```python
from build123d import *

# Parameters (mm, degrees)
SKETCH1_W           = 18.923
SKETCH1_H           = 44.323
BOSS_EXTRUDE1_DEPTH = 63.5
FILLET1_R           = 3.175
SKETCH2_R           = 2.4892
CUT_EXTRUDE1_DEPTH  = 63.5
SKETCH3_R           = 2.4892
CUT_EXTRUDE2_DEPTH  = 63.5


with BuildPart() as part:
    # Sketch1 → Boss-Extrude1 (new body)
    with BuildSketch(Plane.XY):
        with Locations((9.4615, 22.1615)):
            Rectangle(SKETCH1_W, SKETCH1_H)
    extrude(amount=BOSS_EXTRUDE1_DEPTH)

    # Fillet1
    fillet1_edges = [part.edges().sort_by_distance(p)[0] for p in [
        (0, 44.323, 31.75),
        (18.923, 44.323, 31.75),
        (18.923, 0, 31.75),
        (0, 0, 31.75),
    ]]
    fillet(fillet1_edges, radius=FILLET1_R)

    # Sketch2 → Cut-Extrude1 (cut)
    with BuildSketch(Plane(origin=(0, 44.323, 0), x_dir=(1, 0, 0), z_dir=(0, 1, 0))):
        with Locations(Location((9.4615, -6.35, 0), (0, 0, 270))):
            Circle(SKETCH2_R)
        with Locations(Location((9.4615, -19.05, 0), (0, 0, 270))):
            Circle(SKETCH2_R)
        with Locations(Location((9.4615, -31.75, 0), (0, 0, 270))):
            Circle(SKETCH2_R)
        with Locations(Location((9.4615, -44.45, 0), (0, 0, 270))):
            Circle(SKETCH2_R)
        with Locations(Location((9.4615, -57.15, 0), (0, 0, 270))):
            Circle(SKETCH2_R)
    extrude(amount=-CUT_EXTRUDE1_DEPTH, mode=Mode.SUBTRACT)

    # Sketch3 → Cut-Extrude2 (cut)
    with BuildSketch(Plane(origin=(18.923, 0, 0), x_dir=(0, 0, -1), z_dir=(1, 0, 0))):
        with Locations(Location((-57.15, 34.8615, 0), (0, 0, 90))):
            Circle(SKETCH3_R)
        with Locations(Location((-44.45, 34.8615, 0), (0, 0, 90))):
            Circle(SKETCH3_R)
        with Locations(Location((-31.75, 34.8615, 0), (0, 0, 90))):
            Circle(SKETCH3_R)
        with Locations(Location((-19.05, 34.8615, 0), (0, 0, 90))):
            Circle(SKETCH3_R)
        with Locations(Location((-6.35, 34.8615, 0), (0, 0, 90))):
            Circle(SKETCH3_R)
        with Locations(Location((-44.45, 9.4615, 0), (0, 0, 90))):
            Circle(SKETCH3_R)
        with Locations(Location((-31.75, 9.4615, 0), (0, 0, 90))):
            Circle(SKETCH3_R)
        with Locations(Location((-19.05, 9.4615, 0), (0, 0, 90))):
            Circle(SKETCH3_R)
        with Locations(Location((-6.35, 9.4615, 0), (0, 0, 90))):
            Circle(SKETCH3_R)
        with Locations(Location((-57.15, 9.4615, 0), (0, 0, 90))):
            Circle(SKETCH3_R)
    extrude(amount=-CUT_EXTRUDE2_DEPTH, mode=Mode.SUBTRACT)


solid = part.part
```
Could you check a few things on this model? Use its own coordinates, in mm. Round coordinates to 2 decimals unless told otherwise and drop trailing zeros. Write each loop counter-clockwise with the first axis right and the second up, starting at its lowest first coordinate (ties: lowest second). Pieces come first, ordered by that corner, then holes. Notation, with made-up numbers: M 85.5,-23 L 117.5,-23 A22 cw 117.5,8 Z; hole C -24,39 d6. An arc over 180 degrees is marked long. Answer in a Markdown table with one row per item. Add a question column.
Q1. If we mould it in two halves opening along X, with no side actions, what happens to faces 1 (the cylindrical face through (7.95, 40.71, 17.07)), 2 (the cylindrical face through (15.31, 11.836, 7.098)), 3 (the cylindrical face through (0.905, 43.368, 32.194))? For each: +X half, -X half, draft (parallel to the pull), parting line (faces both ways), or undercut.
Q2. Will this pin go through, and if not, where does the flat tip stop? pin 1 Ø6.5 at (x, z) = (9.46, 31.75) entering from +Y.
Q3. Imagine slicing it at A-A (y = 18.5). Please give me the cut outline in (x, z).
Q4. If I drill on line 1 (Y direction, x = 13, z = 31.75); line 2 (X direction, y = 37.5, z = 19.05); line 3 (Y direction, x = 16.25, z = 30), over which ranges is the centre line in solid material (lowest first)? Write a range as from..to.
Q5. Imagine slicing it at C-C (x = 7.75). Give the number of separate pieces and of enclosed holes in the cut face, then the cut area to 3 significant figures.
Q6. Imagine slicing it at B-B (z = 57.15). Please give me the cut outline in (x, y) (3 decimals), then the cut area to 3 significant figures.
Values:
| question | item | result |
|---|---|---|
| 1 | face 1 | undercut |
| 1 | face 2 | draft |
| 1 | face 3 | -X half |
| 2 | pin 1 | y = 44.32 |
| 3 | outline | M 0,0 L 18.92,0 L 18.92,63.5 L 0,63.5 Z; hole C 9.46,6.35 d4.98; hole C 9.46,19.05 d4.98; hole C 9.46,31.75 d4.98; hole C 9.46,44.45 d4.98; hole C 9.46,57.15 d4.98 |
| 4 | line 1 | 0..6.97, 11.95..32.37, 37.35..44.32 |
| 4 | line 2 | 0..6.97, 11.95..18.92 |
| 4 | line 3 | 0.04..7.69, 11.23..33.09, 36.63..44.28 |
| 5 | separate pieces | 6 |
| 5 | enclosed holes | 0 |
| 5 | area | 1,980 mm^2 |
| 6 | outline | M 0,3.175 A3.175 ccw 3.175,0 L 6.972,0 L 6.972,6.972 L 0,6.972 Z; M 0,11.951 L 6.972,11.951 L 6.972,32.372 L 0,32.372 Z; M 0,37.351 L 6.972,37.351 L 6.972,44.323 L 3.175,44.323 A3.175 ccw 0,41.148 Z; M 11.951,0 L 15.748,0 A3.175 ccw 18.923,3.175 L 18.923,6.972 L 11.951,6.972 Z; M 11.951,11.951 L 18.923,11.951 L 18.923,32.372 L 11.951,32.372 Z; M 11.951,37.351 L 18.923,37.351 L 18.923,41.148 A3.175 ccw 15.748,44.323 L 11.951,44.323 Z |
| 6 | area | 471 mm^2 |
